The figure shows three views and two pictorial views of one solid part (mm, origin at its lowest corner). Answer the questions. A direction names the side the tool comes from. Round coordinates to 2 decimals unless told otherwise and drop trailing zeros. Write each loop counter-clockwise with the first axis right and the second up, starting at its lowest first coordinate (ties: lowest second). Pieces come first, ordered by that corner, then holes.
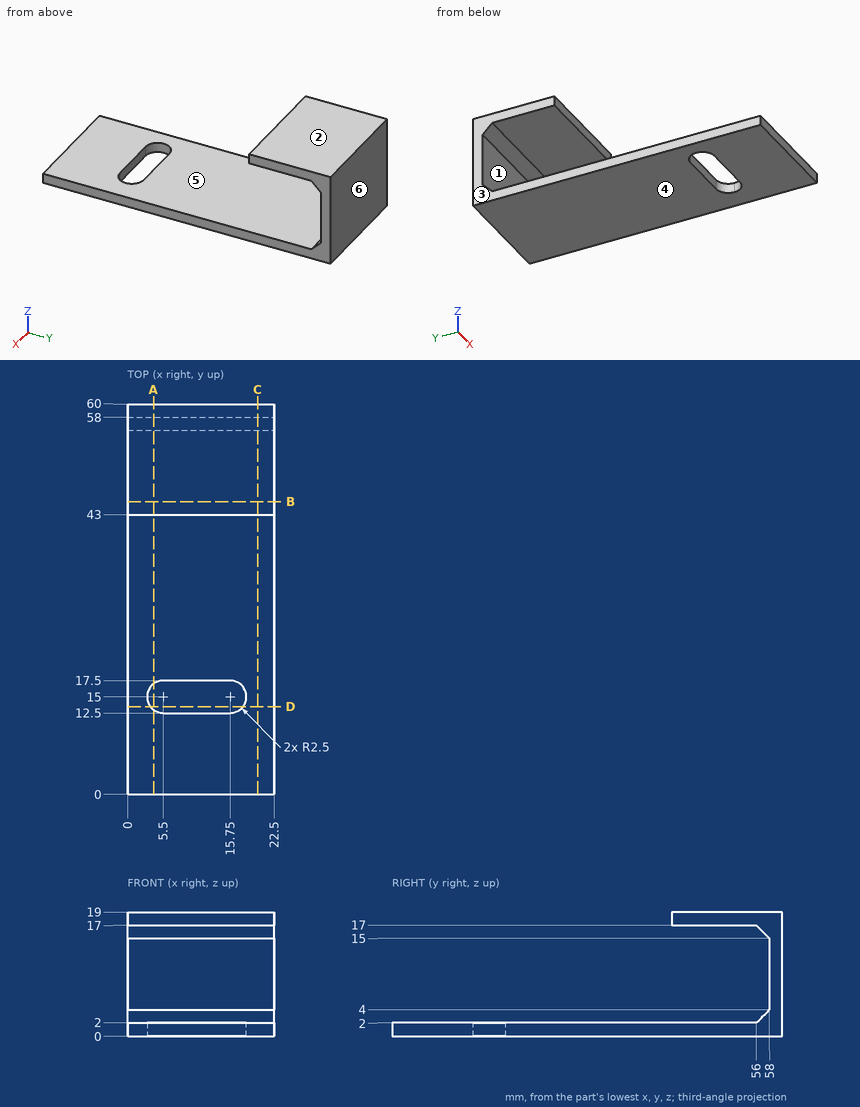
Q1. Section A-A (x = 4) is taken. Determine the outline of the cut face in (y, z), then the cut area to 3 significant figures.
Verdict:
outline: (0, 0) - (13, 0) - (13, 2) - (0, 2) - close; (17, 0) - (60, 0) - (60, 19) - (43, 19) - (43, 17) - (56, 17) - (58, 15) - (58, 4) - (56, 2) - (17, 2) - close
area: 180 mm2
Q2. Straight lines are drawn through the part: probe 1 along Z at (x, y) = (1.5, 44); probe 2 along Y at (x, z) = (17.5, 4.75); probe 3 along Z at (x, y) = (18, 33.5). For each, find the intervals that lie inside material, in ascending order.
Verdict:
probe 1: z = 0 to 2, 17 to 19
probe 2: y = 58 to 60
probe 3: z = 0 to 2
Q3. Which of the six approach directions +Z, -Z, +X, -X, +Y, -Y give full straight-line access (tool end or side, diameter ignored) to the marked faces 5 and 6?
Verdict:
face 5: +X, -X, -Y
face 6: +Z, -Z, +X, -X, +Y
Q4. Section B-B (y = 45) is taken. Determine the outline of the cut face in (x, z).
Verdict:
outline: (0, 0) - (22.5, 0) - (22.5, 2) - (0, 2) - close; (0, 17) - (22.5, 17) - (22.5, 19) - (0, 19) - close
Q5. Flat-ended cylindrical pins translate along their axes: pin 1 Ø10 at (x, y) = (12, 30) entering from +Z; pin 2 Ø1.6 at (x, z) = (13, 18) entering from -Y; pin 3 Ø9 at (x, z) = (9.5, 9.5) entering from -Y. Find the tip coordinate at first contact, or state that the pin passes through.
Verdict:
pin 1: stops at z = 2
pin 2: stops at y = 43
pin 3: stops at y = 58
Q6. Section D-D (y = 13.5) is taken. Determine the outline of the cut face in (x, z), then the cut area to 3 significant figures.
Verdict:
outline: (0, 0) - (3.5, 0) - (3.5, 2) - (0, 2) - close; (17.75, 0) - (22.5, 0) - (22.5, 2) - (17.75, 2) - close
area: 16.5 mm2
Q7. Determine the mould class of the marked faces 1, 2, 3 and 4 for opening direction Z: pulls with the +Z half, pulls with the -Z half, needs draft (parallel to the pull), parting line crosses it, or undercut.
Verdict:
face 1: undercut
face 2: pulls with the +Z half
face 3: needs draft
face 4: pulls with the -Z half
Q8. Section C-C (x = 20) is taken. Determine the outline of the cut face in (y, z).
Verdict:
outline: (0, 0) - (60, 0) - (60, 19) - (43, 19) - (43, 17) - (56, 17) - (58, 15) - (58, 4) - (56, 2) - (0, 2) - close
